```python
from build123d import *

# Parameters (mm, degrees)
F1_DEPTH = 3
F0_R     = 11
F0_R_2   = 7
F2_DEPTH = 10


with BuildPart() as f1:
    # F0 (on Top) → F1 (new body)
    with BuildSketch(Plane.XY):
        with BuildLine():
            ThreePointArc((21, 8), (19.5355339059, 11.5355339059), (16, 13))
            Line((16, 13), (-1.88e-08, 13))
            ThreePointArc((-1.88e-08, 13), (9.1923881488, 9.1923881621), (13, 0))
            ThreePointArc((13, 0), (9.1923881554, -9.1923881554), (0, -13))
            Line((0, -13), (16, -13))
            ThreePointArc((16, -13), (19.5355339059, -11.5355339059), (21, -8))
            Line((21, -8), (21, 8))
        make_face()
    extrude(amount=F1_DEPTH)



with BuildPart() as f1b:
    # F0 (on Top) → F1, piece 2 (new body)
    with BuildSketch(Plane.XY):
        with BuildLine():
            ThreePointArc((0, -13), (-13, -9.4e-09), (-1.88e-08, 13))
            Line((-1.88e-08, 13), (-16, 13))
            ThreePointArc((-16, 13), (-19.5355339059, 11.5355339059), (-21, 8))
            Line((-21, 8), (-21, -8))
            ThreePointArc((-21, -8), (-19.5355339059, -11.5355339059), (-16, -13))
            Line((-16, -13), (0, -13))
        make_face()
    extrude(amount=F1_DEPTH)


with BuildPart() as f1c:
    # F0 (on Top) → F1, piece 3 (new body)
    with BuildSketch(Plane.XY):
        Circle(F0_R)
        Circle(F0_R_2, mode=Mode.SUBTRACT)
    extrude(amount=F1_DEPTH)


with BuildPart() as f1_1:
    add(f1.part)

    add(f1b.part)  # F2 merges F1b

    add(f1c.part)  # F2 merges F1c
    # F0 (on Top) → F2 (join)
    with BuildSketch(Plane.XY):
        with BuildLine():
            ThreePointArc((13, 0), (9.1923881488, 9.1923881621), (-1.88e-08, 13))
            ThreePointArc((-1.88e-08, 13), (-13, -9.4e-09), (0, -13))
            ThreePointArc((0, -13), (9.1923881554, -9.1923881554), (13, 0))
        make_face()
        Circle(F0_R, mode=Mode.SUBTRACT)
    extrude(amount=F2_DEPTH)


solid = f1_1.part
```
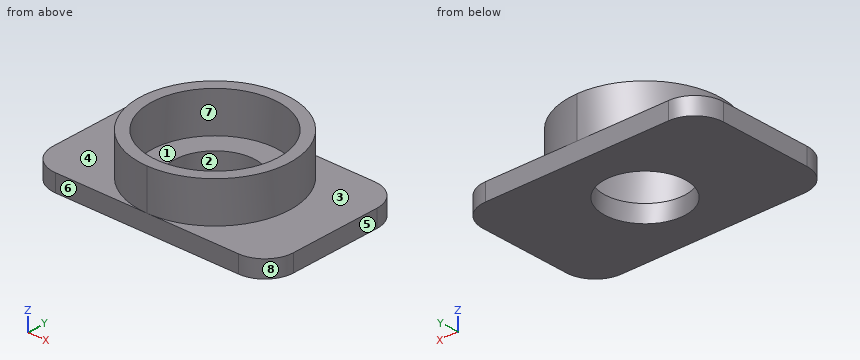
Geometry: final body of the model. Coordinates: model frame, mm. Face numbers are marked on the shaded views. A direction names the side the tool comes from. Round coordinates to 2 decimals unless told otherwise and drop trailing zeros. Order: outer loops, then holes, each group sorted by start corner. A loop starts at its lowest first (then second) coordinate and runs counter-clockwise, first axis right, second up. Notation, with made-up numbers: (-29.5, 73.5) - (-18.5, 73.5) arc R34 cw to (-18.5, 104.5) - close; hole circle Ø10 at (-30, -1.5). An arc over 180 degrees is marked (long way). Use CSV: the item, a comma, the result in double quotes. Start each with the question number.
Q1. Access query for the marked faces 1, 2, 3, 4 and 5. Directions: +Z, -Z, +X, -X, +Y, -Y. A direction counts if a zero-diameter tool reaches every point of the face in a straight line with its end or side. Return the directions, or none.
Q2. Material intervals for line 1 along Y through (x, z) = (0, 6.5); line 2 along Y through (x, z) = (0, 1.8); line 3 along X through (y, z) = (6.25, 3.25), sorted ascending. Write a range as from..to.
Q3. Mould query, pull axis X, two halves, no side actions, for the marked faces 6, 7 and 8. Classes: +X half, -X half, draft (parallel to the pull), parting line (faces both ways), or undercut.
Q4. Section query D-D (y = 9.5). Return loops of the section in (x, z), and give its area (3 significant figures).
Q5. Section query A-A (y = 0). Return loops of the section in (x, z).
Q6. First-contact query: pin 1 (1 mm diameter, centred on x = 5.5, z = 8, fed in from +Y); pin 2 (5 mm diameter, centred on x = -13.5, z = 7, fed in from -Y); pin 3 (4 mm diameter, centred on x = -16.5, z = 6, fed in from +Y); pin 4 (6 mm diameter, centred on x = 10, z = 7.5, fed in from -Y). Flat tips, straight axial feed; report the tip coordinate or a pass-through.
Q7. Section query C-C (z = 5.75). Return loops of the section in (x, y), and give its area (3 significant figures).
Q8. Section query B-B (x = 2.5). Return loops of the section in (y, z), and give its area (3 significant figures).
Result set:
1,face 1,"+Z"
1,face 2,"+Z, -Z"
1,face 3,"+Z, +X"
1,face 4,"+Z, -X"
1,face 5,"+Z, -Z, +X, +Y, -Y"
2,line 1,"y = -13..-11, 11..13"
2,line 2,"y = -13..-7, 7..13"
2,line 3,"x = -11.4..-9.05, 9.05..11.4"
3,face 6,"draft"
3,face 7,"undercut"
3,face 8,"+X half"
4,outline,"(-20.77, 0) - (20.77, 0) - (20.77, 3) - (8.87, 3) - (8.87, 10) - (5.55, 10) - (5.55, 3) - (-5.55, 3) - (-5.55, 10) - (-8.87, 10) - (-8.87, 3) - (-20.77, 3) - close"
4,area,"171 mm2"
5,outline,"(-21, 0) - (-7, 0) - (-7, 3) - (-11, 3) - (-11, 10) - (-13, 10) - (-13, 3) - (-21, 3) - close; (7, 0) - (21, 0) - (21, 3) - (13, 3) - (13, 10) - (11, 10) - (11, 3) - (7, 3) - close"
6,pin 1,"stops at y = 12"
6,pin 2,"stops at y = -6.93"
6,pin 3,"passes through"
6,pin 4,"stops at y = -10.95"
7,outline,"circle Ø26 at (0, 0); hole circle Ø22 at (0, 0)"
7,area,"151 mm2"
8,outline,"(-13, 0) - (-6.54, 0) - (-6.54, 3) - (-10.71, 3) - (-10.71, 10) - (-12.76, 10) - (-12.76, 3) - (-13, 3) - close; (6.54, 0) - (13, 0) - (13, 3) - (12.76, 3) - (12.76, 10) - (10.71, 10) - (10.71, 3) - (6.54, 3) - close"
8,area,"67.4 mm2"
